Autodesk Inventor part; units mm, degrees
ref_plane "YZ Plane" through (0, 0, 0) normal (1, 0, 0) x (0, 1, 0)
ref_plane "XZ Plane" through (0, 0, 0) normal (0, 1, 0) x (-1, 0, 0)
ref_plane "XY Plane" through (0, 0, 0) normal (0, 0, 1) x (1, 0, 0)
sketch "Sketch1" plane through (0, 0, 0) normal (0, 0, 1) x (1, 0, 0)
  line L0 (6, 1.5) -> (6, -1.5)
  line L1 (8, 0.5) -> (11.5, 0.5)
  line L2 (12.5, 1.5) -> (12.5, 2.3)
  line L3 (12.5, 1.5) -> (11.5, 1.5) construction
  line L4 (11.5, 1.5) -> (11.5, 0.5) construction
  arc A0 (11.5, 0.5) -> (12.5, 1.5) centre (11.5, 1.5) ccw
  line L5 (6, 1.5) -> (9.5, 1.5)
  line L6 (12.5, 2.3) -> (9.5, 2.3)
  line L7 (9.5, 2.3) -> (9.5, 1.5)
  line L8 (8, -0.5) -> (8, 0.5)
  line L9 (8, -1.5) -> (8, -0.5)
  line L10 (0, 0) -> (0, 11.9081) construction
  line L11 (8, -1.5) -> (6, -1.5)
  dimension "d0" = 3
  dimension "d1" = 1.5
  dimension "d2" = 0.8
  dimension "d3" = 1
  dimension "d4" = 1
  dimension "d5" = 3
  dimension "d6" = 6
  dimension "d7" = 0.8
  dimension "d8" = 3.5
revolve "Revolution1" add sketch "Sketch1" angle 360 about axis through (0, 0, 0) along (0, 1, 0)
equation "\"d1\" = 0.5 * d0"
equation "\"d4\" = d3"
properties part number "tarcza sprzęgła 2"
Build history of the part. All positions in model axes, mm. A direction names the side the tool comes from. Round coordinates to 2 decimals unless told otherwise and drop trailing zeros. Write each loop counter-clockwise with the first axis right and the second up, starting at its lowest first coordinate (ties: lowest second). Pieces come first, ordered by that corner, then holes. Notation, with made-up numbers: M -11.5,-34 L -2.5,-34 A15 cw -2.5,-13 Z; hole C 72.5,62.25 d9. An arc over 180 degrees is marked long. Answer as a JSON object with one key per item and string values. Group by question number.
(1) Mould opens along Z. For faces 1 (the cylindrical face through (-6, 0, 0)), 2 (the cylindrical face through (11.923, 1.906, -3.755)), 3 (the flat face through (2.7, 2.3, -9.3)) say: pulls with the +Z half, pulls with the -Z half, needs draft (parallel to the pull), parting line crosses it, or undercut.
(2) Drill centre lines: L1, parallel to X at y = -0.6, z = 0; L2, parallel to Z at x = 0, y = 1.8. Where is each one in solid material? Low to high.
(3) Cut at B-B (z = 0). Give the cut face in (x, y), and give its area (3 significant figures).
(4) Which spindle directions (+Z, -Z, +X, -X, +Y, -Y) get a long thin tool onto all of the face, cutting with end or side? Do faces 4 (the flat face through (-2, -1.5, -6)), 5 (the cylindrical face through (-1.73, -0.49, 7.81)), 6 (the cylindrical face through (4.38, 1.89, -8.43)). Say none if no direction does.
(5) Cut at A-A (x = 0). Give the cut face in (y, z), and give its area (3 significant figures).
(6) Flat gauge pins, fed straight in: pin 1 (1 mm diameter, centred on x = -1.5, y = 2, fed in from +Z); pin 2 (9.5 mm diameter, centred on x = 3, z = -2, fed in from +Y); pin 3 (1 mm diameter, centred on y = 1, z = -5.5, fed in from +X). Where does each tip first touch, or does it go through?
Responses:
{
 "1": {"face 1": "undercut", "face 2": "parting line crosses it", "face 3": "needs draft"},
 "2": {"L1": "x = -8 to -6, 6 to 8", "L2": "z = -12.5 to -9.5, 9.5 to 12.5"},
 "3": {"outline": "M -12.5,1.5 A1 ccw -11.5,0.5 L -8,0.5 L -8,-1.5 L -6,-1.5 L -6,1.5 L -9.5,1.5 L -9.5,2.3 L -12.5,2.3 Z; M 6,-1.5 L 8,-1.5 L 8,0.5 L 11.5,0.5 A1 ccw 12.5,1.5 L 12.5,2.3 L 9.5,2.3 L 9.5,1.5 L 6,1.5 Z", "area": "25.4 mm2"},
 "4": {"face 4": "+Z, -Z, +X, -X, -Y", "face 5": "-Y", "face 6": "+Y"},
 "5": {"outline": "M -1.5,-8 L 0.5,-8 L 0.5,-11.5 A1 ccw 1.5,-12.5 L 2.3,-12.5 L 2.3,-9.5 L 1.5,-9.5 L 1.5,-6 L -1.5,-6 Z; M -1.5,6 L 1.5,6 L 1.5,9.5 L 2.3,9.5 L 2.3,12.5 L 1.5,12.5 A1 ccw 0.5,11.5 L 0.5,8 L -1.5,8 Z", "area": "25.4 mm2"},
 "6": {"pin 1": "stops at z = 12.46", "pin 2": "stops at y = 1.5", "pin 3": "stops at x = 11.39"}
}
